```python
from build123d import *

# Parameters (mm, degrees)
SKETCH_1_W          = 76
SKETCH_1_H          = 35
EXTRUDE_1_DEPTH     = 2.5
SKETCH_2_W          = 13
SKETCH_2_H          = 3.5
CUT_EXTRUDE_1_DEPTH = 3.5
SKETCH_3_W          = 3
SKETCH_3_H          = 5.1
SKETCH_3_H_2        = 3.1
SKETCH_3_H_3        = 13.2
CUT_EXTRUDE_2_DEPTH = 3.5
FILLET_1_R          = 1
SKETCH_4_R          = 1.5
SKETCH_4_W          = 9.9
SKETCH_4_H          = 4.5
CUT_EXTRUDE_3_DEPTH = 3.5
SKETCH_5_W          = 10
SKETCH_5_H          = 6
CUT_EXTRUDE_4_DEPTH = 3.5


with BuildPart() as part:
    # 草图1 → 凸台-拉伸1 (new body)
    with BuildSketch(Plane(origin=(0, 0, 0), x_dir=(1, 0, 0), z_dir=(0, 1, 0))):
        Rectangle(SKETCH_1_W, SKETCH_1_H)
    extrude(amount=EXTRUDE_1_DEPTH)

    # 草图2 → 切除-拉伸1 (cut, through all)
    with BuildSketch(Plane(origin=(0, 2.5, 0), x_dir=(1, 0, 0), z_dir=(0, 1, 0))):
        with Locations((-18, -10.75)):
            Rectangle(SKETCH_2_W, SKETCH_2_H)
        with Locations((18, -10.75)):
            Rectangle(SKETCH_2_W, SKETCH_2_H)
    extrude(amount=-CUT_EXTRUDE_1_DEPTH, mode=Mode.SUBTRACT)

    # 草图3 → 切除-拉伸2 (cut, through all)
    with BuildSketch(Plane(origin=(0, 2.5, 0), x_dir=(1, 0, 0), z_dir=(0, 1, 0))):
        with Locations((-36.5, -14.95)):
            Rectangle(SKETCH_3_W, SKETCH_3_H)
        with Locations((-36.5, 15.95)):
            Rectangle(SKETCH_3_W, SKETCH_3_H_2)
        with Locations((-36.5, 1)):
            Rectangle(SKETCH_3_W, SKETCH_3_H_3)
        with Locations((36.5, -14.95)):
            Rectangle(SKETCH_3_W, SKETCH_3_H)
        with Locations((36.5, 1)):
            Rectangle(SKETCH_3_W, SKETCH_3_H_3)
        with Locations((36.5, 15.95)):
            Rectangle(SKETCH_3_W, SKETCH_3_H_2)
    extrude(amount=-CUT_EXTRUDE_2_DEPTH, mode=Mode.SUBTRACT)

    # 圆角1
    fillet_1_edges = [part.edges().sort_by_distance(p)[0] for p in [
        (38, 1.25, -7.6),
        (38, 1.25, 5.6),
        (38, 1.25, -14.4),
        (-38, 1.25, 12.4),
        (-38, 1.25, -14.4),
        (-38, 1.25, 5.6),
        (-38, 1.25, -7.6),
        (38, 1.25, 12.4),
    ]]
    fillet(fillet_1_edges, radius=FILLET_1_R)

    # 草图4 → 切除-拉伸3 (cut, through all)
    with BuildSketch(Plane(origin=(0, 2.5, 0), x_dir=(1, 0, 0), z_dir=(0, 1, 0))):
        with Locations((-30.8, 14.5)):
            Circle(SKETCH_4_R)
        with Locations((21.018135054, 15.25)):
            Rectangle(SKETCH_4_W, SKETCH_4_H)
    extrude(amount=-CUT_EXTRUDE_3_DEPTH, mode=Mode.SUBTRACT)

    # 草图5 → 切除-拉伸4 (cut, through all)
    with BuildSketch(Plane(origin=(0, 2.5, 0), x_dir=(1, 0, 0), z_dir=(0, 1, 0))):
        with Locations((17, -1)):
            Rectangle(SKETCH_5_W, SKETCH_5_H)
    extrude(amount=-CUT_EXTRUDE_4_DEPTH, mode=Mode.SUBTRACT)


solid = part.part
```
Could you check a few things on this model? Use its own coordinates, in mm. A direction names the side the tool comes from. Give positions to 0.01 mm unless a question says otherwise; leave off trailing zeros. Order: outer loops, then holes, each group sorted by start corner. A loop starts at its lowest first (then second) coordinate and runs counter-clockwise, first axis right, second up.
Q1. If I drill on line 1 along X through (y, z) = (1.85, -14.5); line 2 along Z through (x, y) = (-15, 1.65); line 3 along Z through (x, y) = (-30.8, 1.8), over which ranges is the centre line in solid material (lowest first)?
Q2. Suppose I cut it at B-B, the plane x = -30.8. Write out the boundary of the cut face in (y, z).
Q3. Suppose I cut it at C-C, the plane y = 0.4. Count the separate pieces of the cut face and the enclosed holes in it, and give its area (3 significant figures).
Q4. I'm going to push flat-ended pins straight in: P1, Ø6, axis at x = -3, z = -1.5, coming from the -Y side; P2, Ø0.8, axis at y = 0.5, z = 15.5, coming from the -X side; P3, Ø0.6, axis at x = -36, y = 1.5, coming from the -Z side. Where does each tip first touch, or does it pass through?
Q5. Suppose I cut it at D-D, the plane z = 14. Write out the boundary of the cut face in (x, y).
Q6. Suppose I cut it at A-A, the plane z = 3. Write out the boundary of the cut face in (x, y).
Q7. For faces 1 (the flat face through (18, 1, 12.5)), 2 (the flat face through (21, 1, -13)), 3 (the flat face through (-35, 1, 15)), 4 (the flat face through (36, 1, 5.6)), which set-ups out of +Z, -Z, +X, -X, +Y, -Y let a thin tool reach every point of the face, with its end or its side?
Solution:
1. line 1: x = -35 to -32.3, -29.3 to 16.07, 25.97 to 35
1. line 2: z = -17.5 to 9, 12.5 to 17.5
1. line 3: z = -17.5 to -16, -13 to 17.5
2. outline: (0, -17.5) - (2.5, -17.5) - (2.5, -16) - (0, -16) - close; (0, -13) - (2.5, -13) - (2.5, 17.5) - (0, 17.5) - close
3. separate pieces: 1
3. enclosed holes: 4
3. area: 2,330 mm2
4. P1: stops at y = 0
4. P2: stops at x = -35
4. P3: stops at z = -14.4
5. outline: (-35, 0) - (35, 0) - (35, 2.5) - (-35, 2.5) - close
6. outline: (-35, 0) - (12, 0) - (12, 2.5) - (-35, 2.5) - close; (22, 0) - (35, 0) - (35, 2.5) - (22, 2.5) - close
7. face 1: +Y, -Y
7. face 2: -Z, +Y, -Y
7. face 3: +Z, -X, +Y, -Y
7. face 4: +X, +Y, -Y
